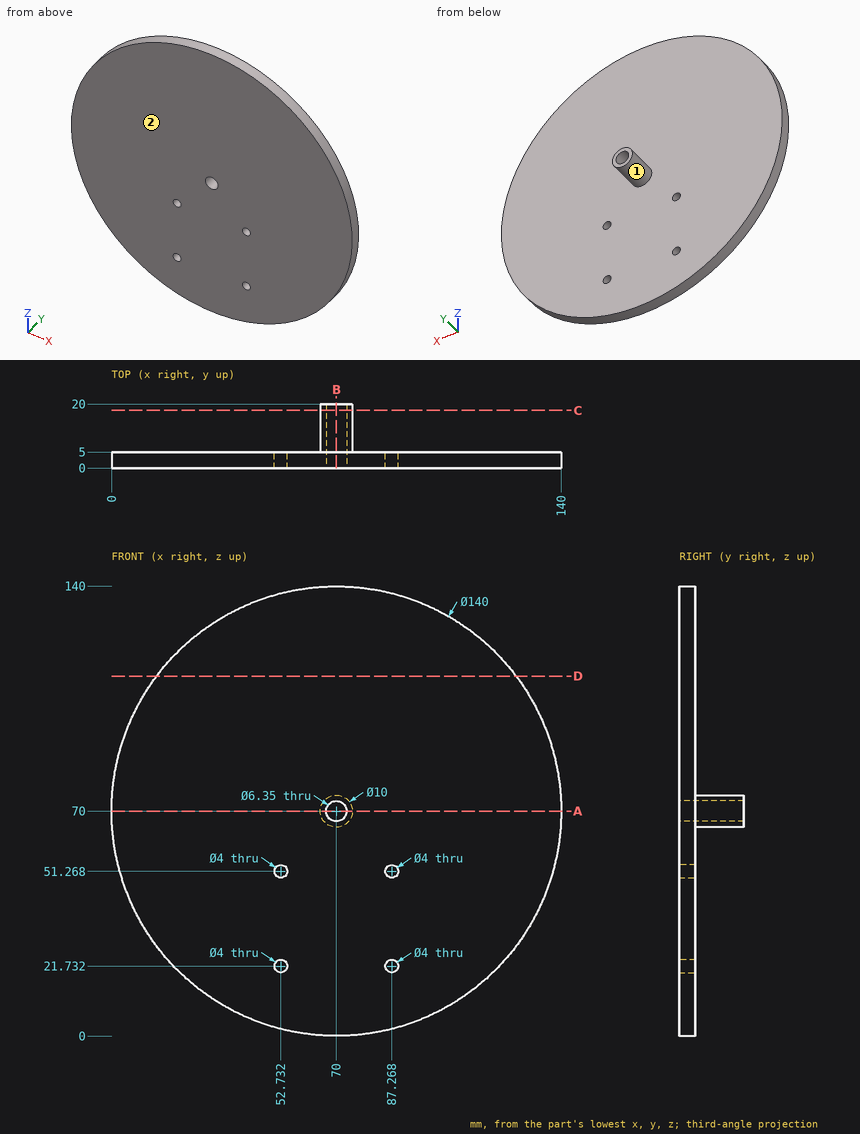
Design review of the part shown in the three views and the two pictorial views. Dimensions are in mm from the part's minimum x, y and z. A direction names the side the tool comes from. Round coordinates to 2 decimals unless told otherwise and drop trailing zeros. Loops run counter-clockwise (first coordinate to the right, second up) from the corner with the lowest first, then second, coordinate; pieces in that order, holes last. Notation, with made-up numbers: (47, 15.25) - (70, 15.25) arc R22 cw to (70, 44.25) - close; hole circle Ø9 at (52.5, -32.75). An arc over 180 degrees is marked (long way). One line per item, written item: value. Start each with the question number.
Item 1: Take a section at B-B (x = 70). Give the boundary of the cut face in (y, z) (3 decimals), plus the area to 3 significant figures.
Item 2: Take a section at A-A (z = 70). Give the boundary of the cut face in (x, y) (3 decimals), plus the area to 3 significant figures.
Item 3: Take a section at D-D (z = 112). Give the boundary of the cut face in (x, y), plus the area to 3 significant figures.
Item 4: For the marked faces 1 and 2, list the 3-axis set-ups (+Z, -Z, +X, -X, +Y, -Y) from which the entire face can be reached by the end or side of a thin tool; tool diameter is ignored.
Item 5: Take a section at C-C (y = 18). Give the boundary of the cut face in (x, z) (3 decimals).
Item 6: For L1, parallel to X at y = 14.75, z = 70 (3 decimals); L2, parallel to X at y = 4.5, z = 72.5 (1 decimal); L3, parallel to Y at x = 105, z = 40.5, list the stretches that pass through material, from the lowest coordinate up.
Item 7: Clearance check with flat-ended pins moving along their axes: pin 1 Ø3 at (x, z) = (96.5, 32.5) entering from -Y; pin 2 Ø6.5 at (x, z) = (87.27, 21.73) entering from +Y. State where each tip first meets the part, or that it passes through.
Answer below:
1. outline: (0, 0) - (5, 0) - (5, 65) - (20, 65) - (20, 66.825) - (0, 66.825) - close; (0, 73.175) - (20, 73.175) - (20, 75) - (5, 75) - (5, 140) - (0, 140) - close
1. area: 723 mm2
2. outline: (0, 0) - (66.825, 0) - (66.825, 20) - (65, 20) - (65, 5) - (0, 5) - close; (73.175, 0) - (140, 0) - (140, 5) - (75, 5) - (75, 20) - (73.175, 20) - close
2. area: 723 mm2
3. outline: (14, 0) - (126, 0) - (126, 5) - (14, 5) - close
3. area: 560 mm2
4. face 1: +Y
4. face 2: +Z, -Z, +X, -X, -Y
5. outline: circle Ø10 at (70, 70); hole circle Ø6.35 at (70, 70)
6. L1: x = 65 to 66.825, 73.175 to 75
6. L2: x = 0 to 68, 72 to 140
6. L3: y = 0 to 5
7. pin 1: stops at y = 0
7. pin 2: stops at y = 5
